```python
from build123d import *

# Parameters (mm, degrees)
BOSS_EXTRUDE1_DEPTH = 10
SKETCH2_R           = 2.5
CUT_EXTRUDE1_DEPTH  = 3


with BuildPart() as part:
    # Sketch1 → Boss-Extrude1 (new body)
    with BuildSketch(Plane.XY):
        Polygon((-27, 38), (-19, 38), (-19, 5), (-14, 0), (14, 0), (19, 5), (19, 38), (27, 38), (27, -3), (22, -8), (-22, -8), (-27, -3), align=None)
    extrude(amount=BOSS_EXTRUDE1_DEPTH)

    # Sketch2 → Cut-Extrude1 (cut)
    with BuildSketch(Plane(origin=(-19, 0, 0), x_dir=(0, 0, -1), z_dir=(1, 0, 0))):
        with Locations(Location((-5, 28.83, 0), (0, 0, 90))):
            Circle(SKETCH2_R)
    extrude(amount=-CUT_EXTRUDE1_DEPTH, mode=Mode.SUBTRACT)


solid = part.part
```
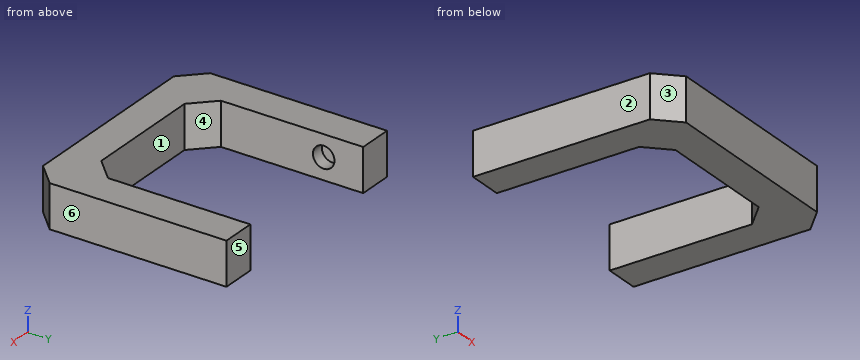
Check sheet for the modelled part. Datum: model origin and axes. Units: mm. Face numbers are marked on the shaded views. A direction names the side the tool comes from. Give positions to 0.01 mm unless a question says otherwise; leave off trailing zeros. Write each loop counter-clockwise with the first axis right and the second up, starting at its lowest first coordinate (ties: lowest second). Pieces come first, ordered by that corner, then holes.
Item 1: Access from +Z, -Z, +X, -X, +Y, -Y to the whole of each face (thin tool, end or side, straight path). Record for the marked faces 1 and 2.
Item 2: Cross-section at D-D (y = 28.83). Enter the section's corners in (x, z), and give its area (3 significant figures).
Item 3: Gauge pin test, flat end, axial feed: pin 1 (1.5 mm diameter, centred on x = -5.5, z = 1.5, fed in from +Y). Record the tip position at first contact, or that the pin passes through.
Item 4: Scan lines: L1, parallel to X at y = 25.5, z = 9.25; L2, parallel to Z at x = -20.9, y = 28.83; L3, parallel to Y at x = -1, z = 4.75. Record each from-to range of solid material in increasing order.
Item 5: Cross-section at B-B (z = 5). Enter the section's corners in (x, y), and give its area (4 significant figures).
Item 6: Cross-section at A-A (y = 15). Enter the section's corners in (x, z), and give its area (3 significant figures).
Item 7: Cross-section at C-C (x = -1). Enter the section's corners in (y, z).
Item 8: Draft check along X on the marked faces 3, 4, 5 and 6. Enter one of: released by +X, released by -X, zero draft, split by the parting line, or undercut.
Report:
1. face 1: +Z, -Z, +Y
1. face 2: +Z, -Z, -X, +Y, -Y
2. outline: (-27, 0) - (-19, 0) - (-19, 2.5) - (-22, 2.5) - (-22, 7.5) - (-19, 7.5) - (-19, 10) - (-27, 10) - close; (19, 0) - (27, 0) - (27, 10) - (19, 10) - close
2. area: 145 mm2
3. pin 1: stops at y = 0
4. L1: x = -27 to -19, 19 to 27
4. L2: z = 0 to 2.5, 7.5 to 10
4. L3: y = -8 to 0
5. outline: (-27, -3) - (-22, -8) - (22, -8) - (27, -3) - (27, 38) - (19, 38) - (19, 5) - (14, 0) - (-14, 0) - (-19, 5) - (-19, 26.33) - (-22, 26.33) - (-22, 31.33) - (-19, 31.33) - (-19, 38) - (-27, 38) - close
5. area: 1,025 mm2
6. outline: (-27, 0) - (-19, 0) - (-19, 10) - (-27, 10) - close; (19, 0) - (27, 0) - (27, 10) - (19, 10) - close
6. area: 160 mm2
7. outline: (-8, 0) - (0, 0) - (0, 10) - (-8, 10) - close
8. face 3: released by -X
8. face 4: undercut
8. face 5: zero draft
8. face 6: released by +X
